For this review, take the finished solid that the model builds, in its own axes (mm). Round coordinates to 2 decimals unless told otherwise and drop trailing zeros. Loops run counter-clockwise (first coordinate to the right, second up) from the corner with the lowest first, then second, coordinate; pieces in that order, holes last.
```python
from build123d import *

# Parameters (mm, degrees)
SKETCH1_R           = 2.05
SKETCH1_R_2         = 11
SKETCH1_R_3         = 6
SKETCH1_R_4         = 7.05
BOSS_EXTRUDE1_DEPTH = 3.175
FILLET1_R           = 2


with BuildPart() as part:
    # Sketch1 → Boss-Extrude1 (new body)
    with BuildSketch(Plane.XY):
        Polygon((88, -24), (88, 24), (48, 24), (-104, 24), (-104, -24), align=None)
        with Locations((-100, -20)):
            Circle(SKETCH1_R, mode=Mode.SUBTRACT)
        with Locations((-8, -16)):
            Circle(SKETCH1_R, mode=Mode.SUBTRACT)
        with Locations((8, -16)):
            Circle(SKETCH1_R, mode=Mode.SUBTRACT)
        Polygon((18, -13), (30, -13), (38.544929421, -20.05), (9.455070579, -20.05), align=None, mode=Mode.SUBTRACT)
        with Locations((84, -20)):
            Circle(SKETCH1_R, mode=Mode.SUBTRACT)
        with Locations((40, -16)):
            Circle(SKETCH1_R, mode=Mode.SUBTRACT)
        Polygon((55.939349424, -19.890566499), (64, -13), (76, -13), (76, -19.706694904), align=None, mode=Mode.SUBTRACT)
        with Locations((60, -8)):
            Circle(SKETCH1_R, mode=Mode.SUBTRACT)
        with Locations((76, -8)):
            Circle(SKETCH1_R, mode=Mode.SUBTRACT)
        Polygon((-38.544929421, 20.05), (-9.455070579, 20.05), (-18, 13), (-30, 13), align=None, mode=Mode.SUBTRACT)
        Polygon((-61.455070579, 20.05), (-70, 13), (-82, 13), (-90.544929421, 20.05), align=None, mode=Mode.SUBTRACT)
        Polygon((-96.991160633, 14.484327085), (-89.991160633, 6), (-89.991160633, -6), (-96.991160633, -14.484327085), align=None, mode=Mode.SUBTRACT)
        Polygon((-90.544929421, -20.05), (-82, -13), (-70, -13), (-61.455070579, -20.05), align=None, mode=Mode.SUBTRACT)
        Polygon((-38.544929421, -20.05), (-30, -13), (-18, -13), (-9.455070579, -20.05), align=None, mode=Mode.SUBTRACT)
        Polygon((-4, -14.484327085), (-11, -6), (-11, 6), (-4, 14.484327085), (4, 14.484327085), (11, 6), (11, -6), (4, -14.484327085), align=None, mode=Mode.SUBTRACT)
        with Locations((-100, 20)):
            Circle(SKETCH1_R, mode=Mode.SUBTRACT)
        with Locations((24, 0)):
            Circle(SKETCH1_R_2, mode=Mode.SUBTRACT)
        Polygon((44, 14.484327085), (48, 9.636140179), (51, 6), (51, -6), (44, -14.484327085), (37, -6), (37, 6), align=None, mode=Mode.SUBTRACT)
        with Locations((68, 0)):
            Circle(SKETCH1_R_3, mode=Mode.SUBTRACT)
        with Locations((60, 8)):
            Circle(SKETCH1_R, mode=Mode.SUBTRACT)
        with Locations((76, 8)):
            Circle(SKETCH1_R, mode=Mode.SUBTRACT)
        with Locations((-8, 16)):
            Circle(SKETCH1_R, mode=Mode.SUBTRACT)
        with Locations((8, 16)):
            Circle(SKETCH1_R, mode=Mode.SUBTRACT)
        Polygon((30, 13), (18, 13), (9.455070579, 20.05), (38.544929421, 20.05), align=None, mode=Mode.SUBTRACT)
        with Locations((40, 16)):
            Circle(SKETCH1_R, mode=Mode.SUBTRACT)
        Polygon((64, 13), (55.939349424, 19.890566499), (76, 19.706694904), (76, 13), align=None, mode=Mode.SUBTRACT)
        with Locations((84, 20)):
            Circle(SKETCH1_R, mode=Mode.SUBTRACT)
        Polygon((-63, 6), (-56, 14.484327085), (-44, 14.484327085), (-37, 6), (-37, -6), (-44, -14.484327085), (-56, -14.484327085), (-63, -6), align=None, mode=Mode.SUBTRACT)
        with Locations((-24, 0)):
            Circle(SKETCH1_R_2, mode=Mode.SUBTRACT)
        with Locations((-40, 16)):
            Circle(SKETCH1_R, mode=Mode.SUBTRACT)
        with Locations((-40, -16)):
            Circle(SKETCH1_R, mode=Mode.SUBTRACT)
        with Locations((-76.495580316, 0)):
            Circle(SKETCH1_R_4, mode=Mode.SUBTRACT)
    extrude(amount=BOSS_EXTRUDE1_DEPTH)

    # Fillet1
    fillet1_edges = [part.edges().sort_by_distance(p)[0] for p in [
        (-44, -14.484327085, 1.5875),
        (-37, -6, 1.5875),
        (-37, 6, 1.5875),
        (-44, 14.484327085, 1.5875),
        (-56, 14.484327085, 1.5875),
        (-63, 6, 1.5875),
        (-63, -6, 1.5875),
        (-56, -14.484327085, 1.5875),
        (76, -19.706694904, 1.5875),
        (76, -13, 1.5875),
        (64, -13, 1.5875),
        (55.939349424, -19.890566499, 1.5875),
        (51, 6, 1.5875),
        (44, 14.484327085, 1.5875),
        (37, 6, 1.5875),
        (37, -6, 1.5875),
        (44, -14.484327085, 1.5875),
        (51, -6, 1.5875),
        (18, 13, 1.5875),
        (30, 13, 1.5875),
        (38.544929421, 20.05, 1.5875),
        (9.455070579, 20.05, 1.5875),
        (9.455070579, -20.05, 1.5875),
        (38.544929421, -20.05, 1.5875),
        (30, -13, 1.5875),
        (18, -13, 1.5875),
        (64, 13, 1.5875),
        (76, 13, 1.5875),
        (76, 19.706694904, 1.5875),
        (55.939349424, 19.890566499, 1.5875),
        (-82, -13, 1.5875),
        (-90.544929421, -20.05, 1.5875),
        (-61.455070579, -20.05, 1.5875),
        (-70, -13, 1.5875),
        (88, -24, 1.5875),
        (-104, -24, 1.5875),
        (-104, 24, 1.5875),
        (88, 24, 1.5875),
        (-61.455070579, 20.05, 1.5875),
        (-90.544929421, 20.05, 1.5875),
        (-82, 13, 1.5875),
        (-70, 13, 1.5875),
        (-30, -13, 1.5875),
        (-38.544929421, -20.05, 1.5875),
        (-9.455070579, -20.05, 1.5875),
        (-18, -13, 1.5875),
        (-11, -6, 1.5875),
        (-4, -14.484327085, 1.5875),
        (4, -14.484327085, 1.5875),
        (11, -6, 1.5875),
        (11, 6, 1.5875),
        (4, 14.484327085, 1.5875),
        (-4, 14.484327085, 1.5875),
        (-11, 6, 1.5875),
        (-18, 13, 1.5875),
        (-9.455070579, 20.05, 1.5875),
        (-38.544929421, 20.05, 1.5875),
        (-30, 13, 1.5875),
        (-96.991160633, 14.484327085, 1.5875),
        (-96.991160633, -14.484327085, 1.5875),
        (-89.991160633, -6, 1.5875),
        (-89.991160633, 6, 1.5875),
    ]]
    fillet(fillet1_edges, radius=FILLET1_R)


solid = part.part
```
(1) Add section C-C (z = 1.7). Give the number of separate pieces and of enclosed holes in the cut face, plus the area to 3 significant figures.
(2) Insertion check: pin 1 Ø11.5 at (x, y) = (-76.5, 0) entering from -Z; pin 2 Ø19 at (x, y) = (68, 0) entering from -Z. Each pin has a flat end and moves straight along its axis. Give the tip position at first contact, or say it passes through.
(3) Add section A-A (x = 24). Give the boundary of the cut face in (y, z) (3 decimals).
(4) For L1, parallel to Y at x = -100, z = 0.85; L2, parallel to Y at x = -39.5, z = 0.6; L3, parallel to Y at x = 24, z = 1.55, list the stretches that pass through material, from the lowest coordinate up.
(5) Add section B-B (x = -8). Give the boundary of the cut face in (y, z) (3 decimals).
Outcome:
1. separate pieces: 1
1. enclosed holes: 32
1. area: 5,410 mm2
2. pin 1: passes through
2. pin 2: stops at z = 0
3. outline: (-24, 0) - (-20.05, 0) - (-20.05, 3.175) - (-24, 3.175) - close; (-13, 0) - (-11, 0) - (-11, 3.175) - (-13, 3.175) - close; (11, 0) - (13, 0) - (13, 3.175) - (11, 3.175) - close; (20.05, 0) - (24, 0) - (24, 3.175) - (20.05, 3.175) - close
4. L1: y = -24 to -22.05, -17.95 to 17.95, 22.05 to 24
4. L2: y = -24 to -17.99, -14.01 to -9.03, 9.03 to 14.01, 17.99 to 24
4. L3: y = -24 to -20.05, -13 to -11, 11 to 13, 20.05 to 24
5. outline: (-24, 0) - (-18.05, 0) - (-18.05, 3.175) - (-24, 3.175) - close; (-13.95, 0) - (-9.636, 0) - (-9.636, 3.175) - (-13.95, 3.175) - close; (9.636, 0) - (13.95, 0) - (13.95, 3.175) - (9.636, 3.175) - close; (18.05, 0) - (24, 0) - (24, 3.175) - (18.05, 3.175) - close
